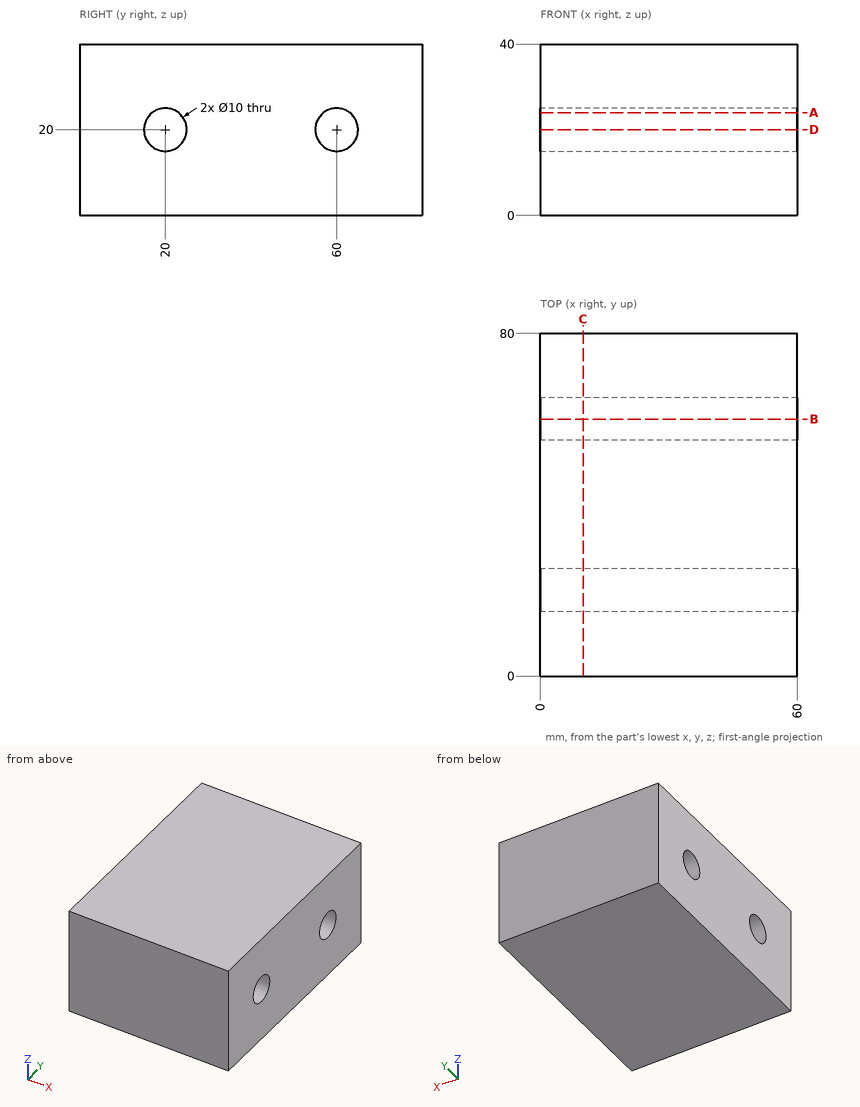
Design review of the part shown in the three views and the two pictorial views. Dimensions are in mm from the part's minimum x, y and z. Round coordinates to 2 decimals unless told otherwise and drop trailing zeros. Write each loop counter-clockwise with the first axis right and the second up, starting at its lowest first coordinate (ties: lowest second). Pieces come first, ordered by that corner, then holes. Notation, with made-up numbers: (3.25, 48.25) - (39.25, 48.25) arc R20 cw to (39.25, 85.25) - close; hole circle Ø7 at (37.25, -23). An arc over 180 degrees is marked (long way). Return JSON: item names as keys, results as strings. Group by question number.
Item 1: We need section B-B on y = 60. Write out the cut boundary in (x, z), and give its area (3 significant figures).
Item 2: We need section D-D on z = 20. Write out the cut boundary in (x, y), and give its area (3 significant figures).
Item 3: We need section A-A on z = 24. Write out the cut boundary in (x, y), and give its area (3 significant figures).
Item 4: We need section C-C on x = 10. Write out the cut boundary in (y, z).
Item 5: For probe 1 along Y at (x, z) = (44.5, 20); probe 2 along Z at (x, y) = (37, 61.5); probe 3 along Y at (x, z) = (39, 15.5), list the stretches that pass through material, from the lowest coordinate up. Write a range as [from, to].
Model answer:
{
 "1": {"outline": "(0, 0) - (60, 0) - (60, 15) - (0, 15) - close; (0, 25) - (60, 25) - (60, 40) - (0, 40) - close", "area": "1,800 mm²"},
 "2": {"outline": "(0, 0) - (60, 0) - (60, 15) - (0, 15) - close; (0, 25) - (60, 25) - (60, 55) - (0, 55) - close; (0, 65) - (60, 65) - (60, 80) - (0, 80) - close", "area": "3,600 mm²"},
 "3": {"outline": "(0, 0) - (60, 0) - (60, 17) - (0, 17) - close; (0, 23) - (60, 23) - (60, 57) - (0, 57) - close; (0, 63) - (60, 63) - (60, 80) - (0, 80) - close", "area": "4,080 mm²"},
 "4": {"outline": "(0, 0) - (80, 0) - (80, 40) - (0, 40) - close; hole circle Ø10 at (20, 20); hole circle Ø10 at (60, 20)"},
 "5": {"probe 1": "y = [0, 15], [25, 55], [65, 80]", "probe 2": "z = [0, 15.23], [24.77, 40]", "probe 3": "y = [0, 17.82], [22.18, 57.82], [62.18, 80]"}
}
